Could you check a few things on this model? Use its own coordinates, in mm. A direction names the side the tool comes from. Give positions to 0.01 mm unless a question says otherwise; leave off trailing zeros. Write each loop counter-clockwise with the first axis right and the second up, starting at its lowest first coordinate (ties: lowest second). Pieces come first, ordered by that corner, then holes. Notation, with made-up numbers: M -23.75,69 L 20.25,69 A24 cw 20.25,95 Z; hole C 20,50.5 d3. An arc over 180 degrees is marked long. One line per item, written item: value.
```python
from build123d import *

# Parameters (mm, degrees)
SKETCH1_W               = 50
SKETCH1_H               = 46
BOSS_EXTRUDE1_DEPTH     = 41
CUT_EXTRUDE1_REACH      = 90.758
SKETCH2_W               = 44
SKETCH2_H               = 40
CUT_EXTRUDE2_DEPTH      = 69.629439747
CUT_EXTRUDE2_DEPTH_BACK = 69.629439747
SKETCH4_W               = 82
SKETCH4_H               = 3
BOSS_EXTRUDE2_DEPTH     = 50
SKETCH7_W               = 16
SKETCH7_H               = 3
BOSS_EXTRUDE4_DEPTH     = 50
SKETCH8_W               = 82
SKETCH8_H               = 46
BOSS_EXTRUDE5_DEPTH     = 3
CUT_EXTRUDE4_START      = -3
CUT_EXTRUDE4_DEPTH      = 103.403219264
CUT_EXTRUDE5_REACH      = 101.403
SKETCH10_W              = 11
SKETCH10_H              = 5
CUT_EXTRUDE6_REACH      = 101.403
SKETCH11_R              = 1.5
SKETCH12_R              = 15
BOSS_EXTRUDE6_DEPTH     = 30
SKETCH13_R              = 12.5
CUT_EXTRUDE7_DEPTH      = 142.063815346
SKETCH14_W              = 2
SKETCH14_H              = 10.8
SKETCH14_H_2            = 13
BOSS_EXTRUDE7_DEPTH     = 68
SKETCH16_R              = 15
BOSS_EXTRUDE8_DEPTH     = 30
CUT_EXTRUDE9_REACH      = 260.917
SKETCH17_R              = 12.5
SKETCH18_W              = 2
SKETCH18_H              = 10.8
BOSS_EXTRUDE9_DEPTH     = 68
SKETCH19_W              = 2
SKETCH19_H              = 13
BOSS_EXTRUDE10_DEPTH    = 68
CUT_EXTRUDE10_REACH     = 160.447
SKETCH15_R              = 2
CUT_EXTRUDE11_REACH     = 160.447
SKETCH20_R              = 2
CUT_EXTRUDE12_REACH     = 160.471
SKETCH21_W              = 50
SKETCH21_H              = 10
CUT_EXTRUDE13_REACH     = 160.471
SKETCH22_W              = 50
SKETCH22_H              = 10


with BuildPart() as part:
    # Sketch1 → Boss-Extrude1 (new, symmetric)
    with BuildSketch(Plane.XY):
        Rectangle(SKETCH1_W, SKETCH1_H)
    extrude(amount=BOSS_EXTRUDE1_DEPTH, both=True)

    # Sketch2 → Cut-Extrude1 (cut, up to next)
    with BuildSketch(Plane.XY.offset(41), mode=Mode.PRIVATE) as cut_extrude1_sk1:
        Rectangle(SKETCH2_W, SKETCH2_H)
    cut_extrude1_tool1 = extrude(cut_extrude1_sk1.sketch, amount=-CUT_EXTRUDE1_REACH, mode=Mode.PRIVATE) & part.part
    add(cut_extrude1_tool1.solids().sort_by_distance((0, 0, 41))[0], mode=Mode.SUBTRACT)

    # Sketch3 → Cut-Extrude2 (cut, two sides: drawn at the far end of the back side and taken through both)
    with BuildSketch(Plane.ZY.offset(25).offset(-CUT_EXTRUDE2_DEPTH_BACK)):
        Polygon((-34, 16), (-34, 20), (34, 20), (34, 16), (38, 16), (38, -16), (34, -16), (34, -20), (-34, -20), (-34, -16), (-38, -16), (-38, 16), align=None)
    extrude(amount=CUT_EXTRUDE2_DEPTH + CUT_EXTRUDE2_DEPTH_BACK, mode=Mode.SUBTRACT)

    # Sketch4 → Boss-Extrude2 (add)
    with BuildSketch(Plane(origin=(25, 0, 0), x_dir=(0, 0, -1), z_dir=(1, 0, 0))):
        with Locations((0, -21.5)):
            Rectangle(SKETCH4_W, SKETCH4_H)
    boss_extrude2 = extrude(amount=BOSS_EXTRUDE2_DEPTH)

    # Sketch7 → Boss-Extrude4 (add)
    with BuildSketch(Plane(origin=(25, 0, 0), x_dir=(0, 0, -1), z_dir=(1, 0, 0))):
        with Locations((0, 21.5)):
            Rectangle(SKETCH7_W, SKETCH7_H)
    boss_extrude4 = extrude(amount=BOSS_EXTRUDE4_DEPTH)

    # Sketch8 → Boss-Extrude5 (add)
    with BuildSketch(Plane(origin=(75, 0, 0), x_dir=(0, 0, -1), z_dir=(1, 0, 0))):
        Rectangle(SKETCH8_W, SKETCH8_H)
    boss_extrude5 = extrude(amount=BOSS_EXTRUDE5_DEPTH)

    # Sketch9 → Cut-Extrude4 (cut)
    with BuildSketch(Plane(origin=(0, 23, 0), x_dir=(1, 0, 0), z_dir=(0, 1, 0)).offset(CUT_EXTRUDE4_START)):
        Polygon((68, -228.237960416), (68, -8), (68, -3), (57, -3), (57, -8), (57, -228.237960416), (57, -668.713881249), (68, -668.713881249), align=None)
    cut_extrude4 = extrude(amount=CUT_EXTRUDE4_DEPTH, mode=Mode.SUBTRACT)

    # Sketch10 → Cut-Extrude5 (cut, up to next)
    with BuildSketch(Plane(origin=(0, 23, 0), x_dir=(1, 0, 0), z_dir=(0, 1, 0)), mode=Mode.PRIVATE) as cut_extrude5_sk1:
        with Locations((37.5, -5.5)):
            Rectangle(SKETCH10_W, SKETCH10_H)
    cut_extrude5_tool1 = extrude(cut_extrude5_sk1.sketch, amount=-CUT_EXTRUDE5_REACH, mode=Mode.PRIVATE) & part.part
    cut_extrude5 = cut_extrude5_tool1.solids().sort_by_distance((37.5, 23, 5.5))[0]
    add(cut_extrude5, mode=Mode.SUBTRACT)

    # Sketch11 → Cut-Extrude6 (cut, up to next)
    with BuildSketch(Plane(origin=(0, 23, 0), x_dir=(1, 0, 0), z_dir=(0, 1, 0)), mode=Mode.PRIVATE) as cut_extrude6_sk1:
        with Locations(Location((29.5, -5.5, 0), (0, 0, 270))):
            Circle(SKETCH11_R)
    cut_extrude6_tool1 = extrude(cut_extrude6_sk1.sketch, amount=-CUT_EXTRUDE6_REACH, mode=Mode.PRIVATE) & part.part
    # Sketch11 → Cut-Extrude6 (cut, up to next)
    with BuildSketch(Plane(origin=(0, 23, 0), x_dir=(1, 0, 0), z_dir=(0, 1, 0)), mode=Mode.PRIVATE) as cut_extrude6_sk2:
        with Locations(Location((45.5, -5.5, 0), (0, 0, 270))):
            Circle(SKETCH11_R)
    cut_extrude6_tool2 = extrude(cut_extrude6_sk2.sketch, amount=-CUT_EXTRUDE6_REACH, mode=Mode.PRIVATE) & part.part
    # Sketch11 → Cut-Extrude6 (cut, up to next)
    with BuildSketch(Plane(origin=(0, 23, 0), x_dir=(1, 0, 0), z_dir=(0, 1, 0)), mode=Mode.PRIVATE) as cut_extrude6_sk3:
        with Locations(Location((54.5, -5.5, 0), (0, 0, 270))):
            Circle(SKETCH11_R)
    cut_extrude6_tool3 = extrude(cut_extrude6_sk3.sketch, amount=-CUT_EXTRUDE6_REACH, mode=Mode.PRIVATE) & part.part
    # Sketch11 → Cut-Extrude6 (cut, up to next)
    with BuildSketch(Plane(origin=(0, 23, 0), x_dir=(1, 0, 0), z_dir=(0, 1, 0)), mode=Mode.PRIVATE) as cut_extrude6_sk4:
        with Locations(Location((70.5, -5.5, 0), (0, 0, 270))):
            Circle(SKETCH11_R)
    cut_extrude6_tool4 = extrude(cut_extrude6_sk4.sketch, amount=-CUT_EXTRUDE6_REACH, mode=Mode.PRIVATE) & part.part
    cut_extrude6_1 = cut_extrude6_tool1.solids().sort_by_distance((29.5, 23, 5.5))[0]
    add(cut_extrude6_1, mode=Mode.SUBTRACT)
    cut_extrude6_2 = cut_extrude6_tool2.solids().sort_by_distance((45.5, 23, 5.5))[0]
    add(cut_extrude6_2, mode=Mode.SUBTRACT)
    cut_extrude6_3 = cut_extrude6_tool3.solids().sort_by_distance((54.5, 23, 5.5))[0]
    add(cut_extrude6_3, mode=Mode.SUBTRACT)
    cut_extrude6_4 = cut_extrude6_tool4.solids().sort_by_distance((70.5, 23, 5.5))[0]
    add(cut_extrude6_4, mode=Mode.SUBTRACT)
    cut_extrude6 = cut_extrude6_1 + cut_extrude6_2 + cut_extrude6_3 + cut_extrude6_4  # Cut-Extrude6 as one shape, for the pattern or mirror that repeats it

    # Sketch12 → Boss-Extrude6 (add)
    with BuildSketch(Plane(origin=(78, 0, 0), x_dir=(0, 0, -1), z_dir=(1, 0, 0))):
        with Locations((26, 0)):
            Circle(SKETCH12_R)
    extrude(amount=BOSS_EXTRUDE6_DEPTH)

    # Sketch13 → Cut-Extrude7 (cut, through all)
    with BuildSketch(Plane(origin=(108, 0, 0), x_dir=(0, 0, -1), z_dir=(1, 0, 0))):
        with Locations((26, 0)):
            Circle(SKETCH13_R)
    extrude(amount=-CUT_EXTRUDE7_DEPTH, mode=Mode.SUBTRACT)

    # Sketch14 → Boss-Extrude7 (add)
    with BuildSketch(Plane(origin=(78, 0, 0), x_dir=(0, 0, -1), z_dir=(1, 0, 0))):
        with Locations((12.3, 17.6)):
            Rectangle(SKETCH14_W, SKETCH14_H)
        with Locations((12.3, -22.5)):
            Rectangle(SKETCH14_W, SKETCH14_H_2)
    extrude(amount=BOSS_EXTRUDE7_DEPTH)

    # Mirror1: Boss-Extrude2, Boss-Extrude4, Boss-Extrude5, Cut-Extrude4, Cut-Extrude5, Cut-Extrude6 across plane
    add(boss_extrude2.mirror(Plane(origin=(0, 0, 0), x_dir=(0, 0, 1), z_dir=(1, 0, 0))))
    add(boss_extrude4.mirror(Plane(origin=(0, 0, 0), x_dir=(0, 0, 1), z_dir=(1, 0, 0))))
    add(boss_extrude5.mirror(Plane(origin=(0, 0, 0), x_dir=(0, 0, 1), z_dir=(1, 0, 0))))
    add(cut_extrude4.mirror(Plane(origin=(0, 0, 0), x_dir=(0, 0, 1), z_dir=(1, 0, 0))), mode=Mode.SUBTRACT)
    add(cut_extrude5.mirror(Plane(origin=(0, 0, 0), x_dir=(0, 0, 1), z_dir=(1, 0, 0))), mode=Mode.SUBTRACT)
    add(cut_extrude6.mirror(Plane(origin=(0, 0, 0), x_dir=(0, 0, 1), z_dir=(1, 0, 0))), mode=Mode.SUBTRACT)

    # Sketch16 → Boss-Extrude8 (add)
    with BuildSketch(Plane.ZY.offset(78)):
        with Locations((26, -1.505120408)):
            Circle(SKETCH16_R)
    extrude(amount=BOSS_EXTRUDE8_DEPTH)

    # Sketch17 → Cut-Extrude9 (cut, up to next)
    with BuildSketch(Plane.ZY.offset(108), mode=Mode.PRIVATE) as cut_extrude9_sk1:
        with Locations((26, -1.505120408)):
            Circle(SKETCH17_R)
    cut_extrude9_tool1 = extrude(cut_extrude9_sk1.sketch, amount=-CUT_EXTRUDE9_REACH, mode=Mode.PRIVATE) & part.part
    add(cut_extrude9_tool1.solids().sort_by_distance((-108, -1.50512, 26))[0], mode=Mode.SUBTRACT)

    # Sketch18 → Boss-Extrude9 (add)
    with BuildSketch(Plane.ZY.offset(78)):
        with Locations((12.3, 17.6)):
            Rectangle(SKETCH18_W, SKETCH18_H)
    extrude(amount=BOSS_EXTRUDE9_DEPTH)

    # Sketch19 → Boss-Extrude10 (add)
    with BuildSketch(Plane.ZY.offset(78)):
        with Locations((12.3, -22.5)):
            Rectangle(SKETCH19_W, SKETCH19_H)
    extrude(amount=BOSS_EXTRUDE10_DEPTH)

    # Sketch15 → Cut-Extrude10 (cut, up to next)
    with BuildSketch(Plane(origin=(0, 0, -13.3), x_dir=(-1, 0, 0), z_dir=(0, 0, -1)), mode=Mode.PRIVATE) as cut_extrude10_sk1:
        with Locations(Location((-143, -24.8, 0), (0, 0, 90))):
            Circle(SKETCH15_R)
    cut_extrude10_tool1 = extrude(cut_extrude10_sk1.sketch, amount=-CUT_EXTRUDE10_REACH, mode=Mode.PRIVATE) & part.part
    # Sketch15 → Cut-Extrude10 (cut, up to next)
    with BuildSketch(Plane(origin=(0, 0, -13.3), x_dir=(-1, 0, 0), z_dir=(0, 0, -1)), mode=Mode.PRIVATE) as cut_extrude10_sk2:
        with Locations(Location((-123, -24.8, 0), (0, 0, 90))):
            Circle(SKETCH15_R)
    cut_extrude10_tool2 = extrude(cut_extrude10_sk2.sketch, amount=-CUT_EXTRUDE10_REACH, mode=Mode.PRIVATE) & part.part
    # Sketch15 → Cut-Extrude10 (cut, up to next)
    with BuildSketch(Plane(origin=(0, 0, -13.3), x_dir=(-1, 0, 0), z_dir=(0, 0, -1)), mode=Mode.PRIVATE) as cut_extrude10_sk3:
        with Locations(Location((-123, 17.2, 0), (0, 0, 90))):
            Circle(SKETCH15_R)
    cut_extrude10_tool3 = extrude(cut_extrude10_sk3.sketch, amount=-CUT_EXTRUDE10_REACH, mode=Mode.PRIVATE) & part.part
    # Sketch15 → Cut-Extrude10 (cut, up to next)
    with BuildSketch(Plane(origin=(0, 0, -13.3), x_dir=(-1, 0, 0), z_dir=(0, 0, -1)), mode=Mode.PRIVATE) as cut_extrude10_sk4:
        with Locations(Location((-143, 17.2, 0), (0, 0, 90))):
            Circle(SKETCH15_R)
    cut_extrude10_tool4 = extrude(cut_extrude10_sk4.sketch, amount=-CUT_EXTRUDE10_REACH, mode=Mode.PRIVATE) & part.part
    add(cut_extrude10_tool1.solids().sort_by_distance((143, -24.8, -13.3))[0], mode=Mode.SUBTRACT)
    add(cut_extrude10_tool2.solids().sort_by_distance((123, -24.8, -13.3))[0], mode=Mode.SUBTRACT)
    add(cut_extrude10_tool3.solids().sort_by_distance((123, 17.2, -13.3))[0], mode=Mode.SUBTRACT)
    add(cut_extrude10_tool4.solids().sort_by_distance((143, 17.2, -13.3))[0], mode=Mode.SUBTRACT)

    # Sketch20 → Cut-Extrude11 (cut, up to next)
    with BuildSketch(Plane.XY.offset(13.3), mode=Mode.PRIVATE) as cut_extrude11_sk1:
        with Locations((-123, 15.694879592)):
            Circle(SKETCH20_R)
    cut_extrude11_tool1 = extrude(cut_extrude11_sk1.sketch, amount=-CUT_EXTRUDE11_REACH, mode=Mode.PRIVATE) & part.part
    # Sketch20 → Cut-Extrude11 (cut, up to next)
    with BuildSketch(Plane.XY.offset(13.3), mode=Mode.PRIVATE) as cut_extrude11_sk2:
        with Locations((-143, 15.694879592)):
            Circle(SKETCH20_R)
    cut_extrude11_tool2 = extrude(cut_extrude11_sk2.sketch, amount=-CUT_EXTRUDE11_REACH, mode=Mode.PRIVATE) & part.part
    # Sketch20 → Cut-Extrude11 (cut, up to next)
    with BuildSketch(Plane.XY.offset(13.3), mode=Mode.PRIVATE) as cut_extrude11_sk3:
        with Locations((-123, -26.305120408)):
            Circle(SKETCH20_R)
    cut_extrude11_tool3 = extrude(cut_extrude11_sk3.sketch, amount=-CUT_EXTRUDE11_REACH, mode=Mode.PRIVATE) & part.part
    # Sketch20 → Cut-Extrude11 (cut, up to next)
    with BuildSketch(Plane.XY.offset(13.3), mode=Mode.PRIVATE) as cut_extrude11_sk4:
        with Locations((-143, -26.305120408)):
            Circle(SKETCH20_R)
    cut_extrude11_tool4 = extrude(cut_extrude11_sk4.sketch, amount=-CUT_EXTRUDE11_REACH, mode=Mode.PRIVATE) & part.part
    add(cut_extrude11_tool1.solids().sort_by_distance((-123, 15.69488, 13.3))[0], mode=Mode.SUBTRACT)
    add(cut_extrude11_tool2.solids().sort_by_distance((-143, 15.69488, 13.3))[0], mode=Mode.SUBTRACT)
    add(cut_extrude11_tool3.solids().sort_by_distance((-123, -26.30512, 13.3))[0], mode=Mode.SUBTRACT)
    add(cut_extrude11_tool4.solids().sort_by_distance((-143, -26.30512, 13.3))[0], mode=Mode.SUBTRACT)

    # Sketch21 → Cut-Extrude12 (cut, up to next)
    with BuildSketch(Plane.XZ.offset(23), mode=Mode.PRIVATE) as cut_extrude12_sk1:
        with Locations((-53, -36)):
            Rectangle(SKETCH21_W, SKETCH21_H)
    cut_extrude12_tool1 = extrude(cut_extrude12_sk1.sketch, amount=-CUT_EXTRUDE12_REACH, mode=Mode.PRIVATE) & part.part
    add(cut_extrude12_tool1.solids().sort_by_distance((-53, -23, -36))[0], mode=Mode.SUBTRACT)

    # Sketch22 → Cut-Extrude13 (cut, up to next)
    with BuildSketch(Plane(origin=(0, -23, 0), x_dir=(-1, 0, 0), z_dir=(0, -1, 0)), mode=Mode.PRIVATE) as cut_extrude13_sk1:
        with Locations((-53, -36)):
            Rectangle(SKETCH22_W, SKETCH22_H)
    cut_extrude13_tool1 = extrude(cut_extrude13_sk1.sketch, amount=-CUT_EXTRUDE13_REACH, mode=Mode.PRIVATE) & part.part
    add(cut_extrude13_tool1.solids().sort_by_distance((53, -23, 36))[0], mode=Mode.SUBTRACT)


solid = part.part
```
1) I'm going to push flat-ended pins straight in: pin 1 (1.5 mm diameter, centred on x = 39.5, y = 22, fed in from +Z); pin 2 (6 mm diameter, centred on x = -104.5, z = 15.5, fed in from -Y); pin 3 (4.5 mm diameter, centred on x = 143, y = -24.8, fed in from +Z); pin 4 (1.8 mm diameter, centred on x = 45.5, z = 5.5, fed in from +Y). Where does each tip first touch, or does it pass through?
Outcome:
pin 1: stops at z = 3
pin 2: stops at y = -29
pin 3: stops at z = -11.3
pin 4: stops at y = -20
2) If we section it at B-B, the plane z = 26: Write out the boundary of the cut face in (x, y).
Outcome:
outline: M -108,-16.51 L -78,-16.51 L -78,-23 L 78,-23 L 78,23 L 75,23 L 75,-20 L -75,-20 L -75,-14.01 L -108,-14.01 Z; M -108,10.99 L -75,10.99 L -75,23 L -78,23 L -78,13.49 L -108,13.49 Z; M -25,20 L 25,20 L 25,23 L -25,23 Z
3) If we section it at A-A, the plane x = 85: Write out the boundary of the cut face in (y, z).
Outcome:
outline: M -29,-13.3 L -16,-13.3 L -16,-11.3 L -29,-11.3 Z; C 0,-26 d30; M 12.2,-13.3 L 23,-13.3 L 23,-11.3 L 12.2,-11.3 Z; hole C 0,-26 d25
4) On a 3-axis mill with a long thin cutter (end or side, diameter ignored), from which of +Z, -Z, +X, -X, +Y, -Y can I reach the whole of each face in a straight line? I mean faces 3 (the face through (-22, 0, -39)), 4 (the face through (112, -23, -13.3)), 5 (the face through (112, -23, -11.3)), 6 (the face through (112, 18, -11.3)), 7 (the face through (-91.731, 6.943, 16.787)). Say none if no direction works.
Outcome:
face 3: +Z, -Z
face 4: -Z, +X, -Y
face 5: +Z, +X, -Y
face 6: +Z, +X, +Y
face 7: -X
5) Please list where these lines run through material, in increasing order: L1, parallel to X at y = 17.2, z = -12.3; L2, parallel to Y at x = -143, z = 12; L3, parallel to X at y = -17.5, z = -0.5. Write a range as from..to.
Outcome:
L1: x = -78..-75, 75..121, 125..141, 145..146
L2: y = -29..-28.31, -24.31..-16, 12.2..13.69, 17.69..23
L3: x = -78..-75, 75..78
6) We'd pull the mould along Y, two halves only. Please class faces 1 (the face through (1, 20, -1)), 2 (the face through (64, -21, 31)): pulls with the +Y half, pulls with the -Y half, needs draft (parallel to the pull), parting line crosses it, or undercut.
Outcome:
face 1: undercut
face 2: needs draft
